Autodesk Inventor part; units mm, degrees
ref_plane "YZ Plane" through (0, 0, 0) normal (1, 0, 0) x (0, 1, 0)
ref_plane "XZ Plane" through (0, 0, 0) normal (0, 1, 0) x (-1, 0, 0)
ref_plane "XY Plane" through (0, 0, 0) normal (0, 0, 1) x (1, 0, 0)
sketch "Sketch1" plane through (0, 0, 0) normal (1, 0, 0) x (0, 1, 0)
  line L0 (-63.3984, -63.5) -> (63.3984, -63.5)
  line L1 (63.3984, -63.5) -> (63.3984, 63.5)
  line L2 (63.3984, 63.5) -> (-63.3984, 63.5)
  line L3 (-63.3984, 63.5) -> (-63.3984, -63.5)
  line L4 (-63.3984, -63.5) -> (63.3984, 63.5) construction
  line L5 (63.3984, -63.5) -> (-63.3984, 63.5) construction
  point P0 (0, 0)
  dimension "d0" = 126.7968
  dimension "d1" = 127
extrude "Extrusion1" add sketch "Sketch1" along normal blind 6.35
sketch "Sketch2" plane through (0, 0, 0) normal (-1, 0, 0) x (0, 0, 1)
  line L0 (60.325, -60.325) -> (-60.325, -60.325)
  line L1 (-60.325, -60.325) -> (-60.325, 60.325)
  line L2 (-60.325, 60.325) -> (60.325, 60.325)
  line L3 (60.325, 60.325) -> (60.325, -60.325)
  line L4 (60.325, -60.325) -> (-60.325, 60.325) construction
  line L5 (-60.325, -60.325) -> (60.325, 60.325) construction
  line L6 (-63.5, -63.3984) -> (-63.5, 63.3984)
  line L7 (63.5, -63.3984) -> (-63.5, -63.3984)
  line L8 (63.5, 63.3984) -> (63.5, -63.3984)
  line L9 (-63.5, 63.3984) -> (63.5, 63.3984)
  line L10 (63.5, 63.3984) -> (-63.5, -63.3984)
  line L11 (63.5, -63.3984) -> (-63.5, -63.3984)
  line L12 (-63.5, 63.3984) -> (63.5, -63.3984)
  point P0 (0, 0)
  point P1 (0, 0)
  point P2 (0, 0)
  dimension "d4" = 120.65
  dimension "d5" = 120.65
extrude "Extrusion2" cut sketch "Sketch2" against normal blind 4.7625 contours L0 L1 L10 L12 L3 | L12 L10 L3 | L1 L12 L10 | L10 L12 L1 L2 L3
sketch "Sketch3" plane through (4.7625, 0, 0) normal (-1, 0, 0) x (0, 0, 1)
  line L0 (57.15, -57.15) -> (-57.15, -57.15)
  line L1 (-57.15, -57.15) -> (-57.15, 57.15)
  line L2 (-57.15, 57.15) -> (57.15, 57.15)
  line L3 (57.15, 57.15) -> (57.15, -57.15)
  line L4 (57.15, -57.15) -> (-57.15, 57.15) construction
  line L5 (-57.15, -57.15) -> (57.15, 57.15) construction
  point P0 (0, 0)
  dimension "d8" = 114.3
  dimension "d9" = 114.3
extrude "Extrusion3" cut sketch "Sketch3" against normal through all
fillet "Fillet1" radius 3.175 8 edges at (2.3813, -60.325, -60.325) (5.5563, -57.15, -57.15) (5.5563, 57.15, 57.15) (5.5563, 57.15, -57.15) (5.5563, -57.15, 57.15) (2.3813, 60.325, 60.325) (2.3813, 60.325, -60.325) (2.3813, -60.325, 60.325)
equation "\"d0\" = width - 2 * alignmentGrooveClearance"
equation "\"d1\" = height"
equation "\"d2\" = plasticThickness"
equation "\"d4\" = height - caseThickness"
equation "\"d5\" = width - caseThickness"
equation "\"d8\" = -caseThickness + height - 2 * mirrorThickness"
equation "\"d9\" = -caseThickness + width - 2 * mirrorThickness"
equation "\"frameAcrylicThickness\" = 9.525"
equation "\"internalAcrylicThickness\" = 6.35"
equation "\"height\" = 127"
equation "\"width\" = 127"
equation "\"depth\" = 203.2"
equation "\"mirrorAngle\" = 2.5deg"
equation "\"detectorWidth\" = 52"
equation "\"detectorHeight\" = 52"
equation "\"mirrorThickness\" = 3.175"
equation "\"fresnelThickness\" = 0.254"
equation "\"focalLength\" = 152.4"
equation "\"ior\" = 1.49"
equation "\"centerThickness\" = 1.27"
equation "\"fresnelAngle\" = 90deg"
equation "\"fresnelEffectiveDiameter\" = 152.4"
equation "\"oRingWidth\" = 1.5875"
equation "\"sensorHolderDepth\" = 19.05"
equation "\"aerogelClearence\" = 3.175"
equation "\"backplanePCBWidth\" = 76.2"
equation "\"backplanePCBHeight\" = 76.2"
equation "\"backplaneHoleOffsett\" = 6.35"
equation "\"backplanePostionOffsett\" = 12.7"
equation "\"moduleSlotClearence\" = 0.79375"
equation "\"aerogelHolderDepth\" = 49.022"
equation "\"plasticThickness\" = 6.35"
equation "\"caseThickness\" = 6.35"
equation "\"alignmantGrooveDepth\" = 1.5875"
equation "\"alignmentGrooveDepth\" = 1.5875"
equation "\"alignmentGrooveClearance\" = 0.1016"
equation "\"frontPanelThickness\" = 1.5875"
equation "\"fresnelGrooveWidth\" = 1.778"
properties part number "mirrorFrontFrame" material "ABS Plastic"
Design review of the part built by this model. Coordinates are the model's own, in mm. A direction names the side the tool comes from. Coordinates: 2 decimals unless noted, no trailing zeros. Order: outer loops, then holes, each group sorted by start corner. A loop starts at its lowest first (then second) coordinate and runs counter-clockwise, first axis right, second up. Notation, with made-up numbers: (-13, -9) -> (23, -9) arc R25 cw to (23, 27) -> close; hole circle Ø7 at (-36.5, 12.5). An arc over 180 degrees is marked (long way). One line per item, written item: value. Start each with the question number.
Q1. Mouldability with a two-part tool opening along Y and no side actions: class faces 1 (the flat face through (3, 63.398, -1)), 2 (the flat face through (6.35, -61, 0)), 3 (the cylindrical face through (5.57, -56.2, 56.24)) as pulls with the +Y half, pulls with the -Y half, needs draft (parallel to the pull), parting line crosses it, or undercut.
Q2. Tool access review of faces 4 (the flat face through (3, -63.398, 1)), 5 (the cylindrical face through (5.57, 56.2, -56.24)), 6 (the flat face through (4.762, -58, -5)): name each direction out of +Z, -Z, +X, -X, +Y, -Y from which nothing blocks a thin tool from reaching the whole face with its end or side.
Q3. For probe 1 along Y at (x, z) = (1, 56) (3 decimals); probe 2 along Y at (x, z) = (6, 38.5); probe 3 along Z at (x, y) = (0.75, 41.5) (3 decimals), list the stretches that pass through material, from the lowest coordinate up.
Q4. Take a section at C-C, the plane x = 1.5. State the section outline as (y, z) points (3 decimals), then the cut area to 3 significant figures.
Values follow:
1. face 1: pulls with the +Y half
1. face 2: needs draft
1. face 3: undercut
2. face 4: +Z, -Z, +X, -X, -Y
2. face 5: +X, -X
2. face 6: -X
3. probe 1: y = -63.398 to -60.325, 60.325 to 63.398
3. probe 2: y = -63.4 to -57.15, 57.15 to 63.4
3. probe 3: z = -63.5 to -60.325, 60.325 to 63.5
4. outline: (-63.398, -63.5) -> (63.398, -63.5) -> (63.398, 63.5) -> (-63.398, 63.5) -> close; hole (-60.325, -57.15) arc R3.175 ccw to (-57.15, -60.325) -> (57.15, -60.325) arc R3.175 ccw to (60.325, -57.15) -> (60.325, 57.15) arc R3.175 ccw to (57.15, 60.325) -> (-57.15, 60.325) arc R3.175 ccw to (-60.325, 57.15) -> close
4. area: 1,560 mm2
